Input: part model. Units: mm. Frame: model coordinates. A direction names the side the tool comes from. Coordinates: 2 decimals unless noted, no trailing zeros. Loops run counter-clockwise (first coordinate to the right, second up) from the corner with the lowest first, then second, coordinate; pieces in that order, holes last.
(1) Line query: L1, parallel to Z at x = -3.75, y = 45.5; L2, parallel to X at y = 2.4, z = -25; L3, parallel to Z at x = -3.25, y = 50.5. Output: solid intervals per line, ascending.
(2) Section B-B, the plane y = 34. Return loops of the section in (x, z).
(3) Section D-D, the plane x = -9.5. Return loops of the section in (y, z), then the cut area to 3 significant figures.
(4) Set-up query: faces 1 (the face through (0, 28, 18.762)), 2 (the face through (0, 19, 0)), 3 (the face through (-1.5, 15.1, -1.3)). Return all of +Z, -Z, +X, -X, +Y, -Y with unobstructed straight access to the full face (end or side cutting, diameter ignored); none if empty.
(5) Section C-C, the plane z = 25. Return loops of the section in (x, y), then the cut area to 3 significant figures.
(6) Contact query for flat-ended pins moving along their axis: P1, Ø1.5, axis at x = 6.5, y = 17, coming from the -Z side; P2, Ø3.5, axis at x = 3.5, z = -23.5, coming from the +Y side; P3, Ø7, axis at x = 4.5, y = 40, coming from the +Z side. Output: stop coordinate, or through.
(7) Mould query, pull axis Y, two halves, no side actions, for faces 4 (the face through (0, 3, -23)), 5 (the face through (0, 18, 11)), 6 (the face through (0, 2, 31.026)), 7 (the face through (-6, 16, 0)). Classes: released by +Y, released by -Y, zero draft, split by the parting line, or undercut.
(8) Section A-A, the plane x = 0. Return loops of the section in (y, z).
```python
from build123d import *

# Parameters (mm, degrees)
SKETCH3_W           = 13.566130208
SKETCH3_H           = 6
BOSS_EXTRUDE1_DEPTH = 11.5
SKETCH4_R           = 1.5
CUT_EXTRUDE1_DEPTH  = 11.5
SKETCH5_W           = 75.75040558
SKETCH5_H           = 1
CUT_EXTRUDE2_DEPTH  = 26
BOSS_EXTRUDE2_DEPTH = 11.5


with BuildPart() as part:
    # Sketch2 → Revolve1 (revolve)
    with BuildSketch(Plane(origin=(0, 0, 0), x_dir=(1, 0, 0), z_dir=(0, 1, 0)), mode=Mode.PRIVATE) as revolve1_sk:
        Polygon((-11.5, 16), (-1.5, 16), (-1.5, 15), (1.5, 15), (1.5, 16), (11.5, 16), (11.5, 19), (-11.5, 19), align=None)
    revolve(revolve1_sk.sketch.rotate(Axis((-71.722155375, 0, 0), (1, 0, 0)), 180), axis=Axis((-71.722155375, 0, 0), (1, 0, 0)))

    # Sketch3 → Boss-Extrude1 (add, symmetric)
    with BuildSketch(Plane(origin=(0, 0, 0), x_dir=(0, 0, -1), z_dir=(1, 0, 0))):
        with Locations((24.243185686, 0)):
            Rectangle(SKETCH3_W, SKETCH3_H)
        with Locations((-24.243185686, 0)):
            Rectangle(SKETCH3_W, SKETCH3_H)
    extrude(amount=BOSS_EXTRUDE1_DEPTH, both=True)

    # Sketch4 → Cut-Extrude1 (cut, symmetric)
    with BuildSketch(Plane(origin=(0, 0, 0), x_dir=(1, 0, 0), z_dir=(0, 1, 0))):
        with Locations(Location((0, 25, 0), (0, 0, 270))):
            Circle(SKETCH4_R)
        with Locations(Location((0, -25, 0), (0, 0, 270))):
            Circle(SKETCH4_R)
    extrude(amount=CUT_EXTRUDE1_DEPTH, both=True, mode=Mode.SUBTRACT)

    # Sketch5 → Cut-Extrude2 (cut, symmetric)
    with BuildSketch(Plane(origin=(0, 0, 0), x_dir=(0, 0, -1), z_dir=(1, 0, 0))):
        Rectangle(SKETCH5_W, SKETCH5_H)
    extrude(amount=CUT_EXTRUDE2_DEPTH, both=True, mode=Mode.SUBTRACT)


with BuildPart() as cut_extrude2_piece_1:
    # of the separate pieces the step leaves, piece 1, a body of its own (cut_extrude2_pieces)
    add(part.part.solids().sort_by_distance((-11.5, 0.5, -15.992185592))[0])

    # Sketch7 → Boss-Extrude2 (add, symmetric)
    with BuildSketch(Plane(origin=(0, 0, 0), x_dir=(0, 0, -1), z_dir=(1, 0, 0))):
        with BuildLine():
            Line((-18.761663039, 53), (-18.761663039, 3))
            ThreePointArc((-18.761663039, 3), (-14.510732941, 12.265342618), (-6.08276253, 18))
            Line((-6.08276253, 18), (-16, 18))
            Line((-16, 18), (-16, 50))
            Line((-16, 50), (16, 50))
            Line((16, 50), (16, 18))
            Line((16, 18), (6.08276253, 18))
            ThreePointArc((6.08276253, 18), (14.510732941, 12.265342618), (18.761663039, 3))
            Line((18.761663039, 3), (18.761663039, 53))
            Line((18.761663039, 53), (-18.761663039, 53))
        make_face()
    extrude(amount=BOSS_EXTRUDE2_DEPTH, both=True)


with BuildPart() as cut_extrude2_piece_2:
    # of the separate pieces the step leaves, piece 2, a body of its own (cut_extrude2_pieces)
    add(part.part.solids().sort_by_distance((-11.5, -0.5, 15.992185592))[0])


solid = cut_extrude2_piece_1.part
```
Report:
1. L1: z = -18.76 to -16, 16 to 18.76
1. L2: x = -11.5 to -1.5, 1.5 to 11.5
1. L3: z = -18.76 to 18.76
2. outline: (-11.5, -18.76) - (11.5, -18.76) - (11.5, -16) - (-11.5, -16) - close; (-11.5, 16) - (11.5, 16) - (11.5, 18.76) - (-11.5, 18.76) - close
3. outline: (0.5, -31.03) - (3, -31.03) - (3, -18.76) - (53, -18.76) - (53, 18.76) - (3, 18.76) - (3, 31.03) - (0.5, 31.03) - (0.5, 15.99) arc R16 cw to (0.5, -15.99) - close; hole (18, -16) - (50, -16) - (50, 16) - (18, 16) - (18, 6.08) arc R19 cw to (18, -6.08) - close
3. area: 629 mm2
4. face 1: +Z, +X, -X, +Y
4. face 2: +X, -X
4. face 3: -X, -Y
5. outline: (-11.5, 0.5) - (-1.5, 0.5) - (-1.5, 3) - (-11.5, 3) - close; (1.5, 0.5) - (11.5, 0.5) - (11.5, 3) - (1.5, 3) - close
5. area: 50.0 mm2
6. P1: stops at z = -18.76
6. P2: stops at y = 3
6. P3: stops at z = 18.76
7. face 4: released by +Y
7. face 5: undercut
7. face 6: zero draft
7. face 7: released by -Y
8. outline: (0.5, -31.03) - (3, -31.03) - (3, -26.5) - (0.5, -26.5) - close; (0.5, -23.5) - (3, -23.5) - (3, -18.76) - (53, -18.76) - (53, 18.76) - (3, 18.76) - (3, 23.5) - (0.5, 23.5) - (0.5, 14.99) arc R15 cw to (0.5, -14.99) - close; (0.5, 26.5) - (3, 26.5) - (3, 31.03) - (0.5, 31.03) - close; hole (18, -16) - (50, -16) - (50, 16) - (18, 16) - (18, 6.08) arc R19 cw to (18, -6.08) - close
